from build123d import *

# Parameters (mm, degrees)
SKETCH_1_W      = 85
SKETCH_1_H      = 40
SKETCH_1_R      = 2.25
SKETCH_1_R_2    = 2
EXTRUDE_1_DEPTH = 3


with BuildPart() as part:
    # 草图1 → 凸台-拉伸1 (new body)
    with BuildSketch(Plane.XY):
        with Locations((20.25, 0)):
            Rectangle(SKETCH_1_W, SKETCH_1_H)
        with Locations((15.25, 13)):
            Circle(SKETCH_1_R, mode=Mode.SUBTRACT)
        with Locations((15.25, -13)):
            Circle(SKETCH_1_R, mode=Mode.SUBTRACT)
        with Locations((57, 15)):
            Circle(SKETCH_1_R_2, mode=Mode.SUBTRACT)
        with Locations((38, 15)):
            Circle(SKETCH_1_R_2, mode=Mode.SUBTRACT)
        with Locations(Location((57, -15, 0), (0, 0, 180))):
            Circle(SKETCH_1_R_2, mode=Mode.SUBTRACT)
        with Locations(Location((38, -15, 0), (0, 0, 180))):
            Circle(SKETCH_1_R_2, mode=Mode.SUBTRACT)
        with BuildLine():
            Line((-14.25, 10.75), (-16.25, 10.75))
            ThreePointArc((-16.25, 10.75), (-18.5, 13), (-16.25, 15.25))
            Line((-16.25, 15.25), (-14.25, 15.25))
            ThreePointArc((-14.25, 15.25), (-12, 13), (-14.25, 10.75))
        make_face(mode=Mode.SUBTRACT)
        with BuildLine():
            Line((-14.25, -15.25), (-16.25, -15.25))
            ThreePointArc((-16.25, -15.25), (-18.5, -13), (-16.25, -10.75))
            Line((-16.25, -10.75), (-14.25, -10.75))
            ThreePointArc((-14.25, -10.75), (-12, -13), (-14.25, -15.25))
        make_face(mode=Mode.SUBTRACT)
        with BuildLine():
            Line((42.5, -12.5), (42.5, 12.5))
            ThreePointArc((42.5, 12.5), (45, 15), (47.5, 12.5))
            Line((47.5, 12.5), (47.5, -12.5))
            ThreePointArc((47.5, -12.5), (45, -15), (42.5, -12.5))
        make_face(mode=Mode.SUBTRACT)
    extrude(amount=EXTRUDE_1_DEPTH)


solid = part.part
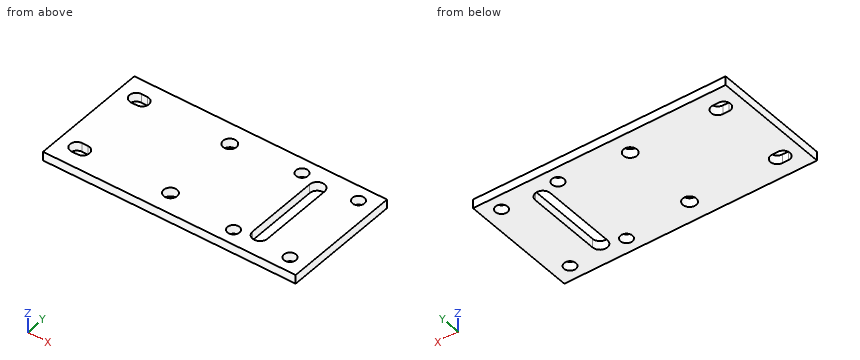
The model under review builds one solid part; all positions refer to its coordinate system, in mm. Coordinates: 2 decimals unless noted, no trailing zeros. Write each loop counter-clockwise with the first axis right and the second up, starting at its lowest first coordinate (ties: lowest second). Pieces come first, ordered by that corner, then holes. Notation, with made-up numbers: (45.25, -5.75) - (51.25, -5.75) arc R15 cw to (51.25, 19.25) - close; hole circle Ø5 at (58.5, 58). An arc over 180 degrees is marked (long way). Answer as a JSON object with one key per item and string values. Group by question number.
1. Clearance check with a flat-ended pin moving along its axis: pin 1 Ø4 at (x, y) = (15.25, 13) entering from +Z. State where the tip first meets the part, or that it passes through.
2. Add section B-B (x = 38). Give the boundary of the cut face in (y, z), plus the area to 3 significant figures.
3. To check wall thickness, follow probe 1 along Y at (x, z) = (38, 2.6); probe 2 along X at (y, z) = (-5, 1.5); probe 3 along Y at (x, z) = (-14.5, 0.95). State the ranges of each line that lie inside material, in increasing order.
4. Add section A-A (y = -9). Give the boundary of the cut face in (x, z).
5. Add section C-C (z = 1.4). Give the number of separate pieces and of enclosed holes in the cut face, plus the area to 3 significant figures.
Findings:
{
 "1": {"pin 1": "through"},
 "2": {"outline": "(-20, 0) - (-17, 0) - (-17, 3) - (-20, 3) - close; (-13, 0) - (13, 0) - (13, 3) - (-13, 3) - close; (17, 0) - (20, 0) - (20, 3) - (17, 3) - close", "area": "96.0 mm²"},
 "3": {"probe 1": "-20 to -17, -13 to 13, 17 to 20", "probe 2": "-22.25 to 42.5, 47.5 to 62.75", "probe 3": "-20 to -15.25, -10.75 to 10.75, 15.25 to 20"},
 "4": {"outline": "(-22.25, 0) - (42.5, 0) - (42.5, 3) - (-22.25, 3) - close; (47.5, 0) - (62.75, 0) - (62.75, 3) - (47.5, 3) - close"},
 "5": {"separate pieces": "1", "enclosed holes": "9", "area": "3,120 mm²"}
}
